from build123d import *


with BuildPart() as part:
    # Esquisse1 → Base-Révolution (revolve)
    with BuildSketch(Plane.XY, mode=Mode.PRIVATE) as base_r_volution_sk:
        with BuildLine():
            Line((1.5, 6), (28.5, 6))
            ThreePointArc((28.5, 6), (29.560660172, 5.560660172), (30, 4.5))
            Line((30, 4.5), (30, 4))
            Line((30, 4), (29, 4))
            Line((29, 4), (29, 4.5))
            ThreePointArc((29, 4.5), (28.853553391, 4.853553391), (28.5, 5))
            Line((28.5, 5), (1.5, 5))
            ThreePointArc((1.5, 5), (1.146446609, 4.853553391), (1, 4.5))
            Line((1, 4.5), (1, 4))
            Line((1, 4), (0, 4))
            Line((0, 4), (0, 4.5))
            ThreePointArc((0, 4.5), (0.439339828, 5.560660172), (1.5, 6))
        make_face()
    revolve(base_r_volution_sk.sketch.rotate(Axis((0, 0, 0), (1, 0, 0)), 90), axis=Axis((0, 0, 0), (1, 0, 0)))


solid = part.part
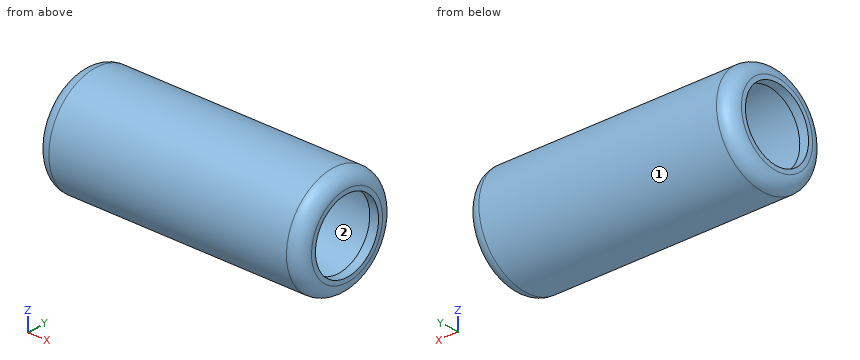
Model file for the job. Use its own axes, mm. Face numbers are marked on the shaded views. Round coordinates to 2 decimals unless told otherwise and drop trailing zeros. Loops run counter-clockwise (first coordinate to the right, second up) from the corner with the lowest first, then second, coordinate; pieces in that order, holes last. Notation, with made-up numbers: (-38, -28.75) -> (0, -28.75) arc R23 ccw to (0, 2.25) -> close; hole circle Ø2 at (83, 72). An arc over 180 degrees is marked (long way). Answer as CSV lines item,"result". Start each with the question number.
1) Pin check, flat tips, straight feed: P1, Ø4, axis at x = 11, y = 2.5, coming from the -Z side; P2, Ø3, axis at y = -0.5, z = -0.5, coming from the +X side; P3, Ø5, axis at x = 18.5, z = 3.5, coming from the +Y side; P4, Ø1.5, axis at x = 8.5, y = 4.5, coming from the -Z side. Stop position of each tip, or through.
2) Slice it at C-C (x = 5). List the corners of the cut face in (y, z).
3) Probe line 1 along X through (y, z) = (-4, 1); line 2 along Y through (x, z) = (28, 0); line 3 along Z through (x, y) = (5, 0.5). List the from-to ranges inside material, lowest first.
4) Mould opens along X. For the marked faces 1 and 2 say: +X half, -X half, draft (parallel to the pull), parting line (faces both ways), or undercut.
5) Slice it at A-A (z = 0). List the corners of the cut face in (x, y).
Filled in:
1,P1,"stops at z = -5.98"
1,P2,"passes through"
1,P3,"stops at y = 5.92"
1,P4,"stops at z = -4.68"
2,outline,"circle Ø12 at (0, 0); hole circle Ø10 at (0, 0)"
3,line 1,"x = 0 to 1, 29 to 30"
3,line 2,"y = -6 to -5, 5 to 6"
3,line 3,"z = -5.98 to -4.97, 4.97 to 5.98"
4,face 1,"draft"
4,face 2,"undercut"
5,outline,"(0, -4.5) arc R1.5 ccw to (1.5, -6) -> (28.5, -6) arc R1.5 ccw to (30, -4.5) -> (30, -4) -> (29, -4) -> (29, -4.5) arc R0.5 cw to (28.5, -5) -> (1.5, -5) arc R0.5 cw to (1, -4.5) -> (1, -4) -> (0, -4) -> close; (0, 4) -> (1, 4) -> (1, 4.5) arc R0.5 cw to (1.5, 5) -> (28.5, 5) arc R0.5 cw to (29, 4.5) -> (29, 4) -> (30, 4) -> (30, 4.5) arc R1.5 ccw to (28.5, 6) -> (1.5, 6) arc R1.5 ccw to (0, 4.5) -> close"
